Read the model definition and answer for the solid it produces. Units are mm, in the model's axes. Face numbers are marked on the shaded views. Coordinates: 2 decimals unless noted, no trailing zeros. Loops run counter-clockwise (first coordinate to the right, second up) from the corner with the lowest first, then second, coordinate; pieces in that order, holes last.
Q1. Section B-B (x = -25.4) is taken. Give the vertices of the cut face in (y, z).
Q2. Section C-C (y = 4.75) is taken. Give the vertices of the cut face in (x, z) (3 decimals), then the cut area to 3 significant figures.
Q3. Straight lines are drawn through the part: line 1 (Z direction, x = 0, y = 1.25); line 2 (Z direction, x = -25, y = 0); line 3 (X direction, y = -1, z = -16.5). For each, find the intervals that lie inside material, in ascending order.
Q4. The mould has two halves that part along X. Classify the marked faces 1, 2 and 3: pulls with the +X half, pulls with the -X half, needs draft (parallel to the pull), parting line crosses it, or undercut.
Q5. Flat-ended cylindrical pins translate along their axes: P1, Ø7.5, axis at x = -24.892, z = 0, coming from the +Y side; P2, Ø2, axis at y = 2.5, z = -4, coming from the +X side. Find the tip coordinate at first contact, or state that the pin passes through.
Q6. Section A-A (z = 2) is taken. Give the vertices of the cut face in (x, y).
from build123d import *

# Parameters (mm, degrees)
F0_W        = 88.9
F0_H        = 63.5
F0_R        = 3.175
F1_DEPTH    = 6.35
F2_R        = 3.81
F3_DEPTH    = 25.4
F4_T1_DEPTH = 88.9
F4_T3_DEPTH = 114.3


# Not quite as in the source:
# - a fillet or chamfer that OpenCascade refuses, or shapes differently, is made with other operations: its cross-section is extruded or revolved along the edge and cut away or added


with BuildPart() as f1:
    # F0 (on Front) → F1 (new body, symmetric)
    with BuildSketch(Plane.XZ):
        Rectangle(F0_W, F0_H)
        with Locations((0, -24.892)):
            Circle(F0_R, mode=Mode.SUBTRACT)
        with BuildLine():
            ThreePointArc((-21.717, 0), (-24.892, -3.175), (-28.067, 0))
            ThreePointArc((-28.067, 0), (-24.892, 3.175), (-21.717, 0))
        make_face(mode=Mode.SUBTRACT)
        with Locations((24.892, 0)):
            Circle(F0_R, mode=Mode.SUBTRACT)
        with BuildLine():
            ThreePointArc((0, 21.717), (-3.175, 24.892), (0, 28.067))
            ThreePointArc((0, 28.067), (2.2450640303, 27.1370640303), (3.175, 24.892))
            ThreePointArc((3.175, 24.892), (2.2450640303, 22.6469359697), (0, 21.717))
        make_face(mode=Mode.SUBTRACT)
    extrude(amount=F1_DEPTH, both=True)

    # F2 (on face) → F3 (cut)
    with BuildSketch(Plane(origin=(0, 0, -31.75), x_dir=(1, 0, 0), z_dir=(0, 0, -1))):
        with Locations((-25.4, 0)):
            Circle(F2_R)
        with BuildLine():
            ThreePointArc((29.21, 0), (25.4, 3.81), (21.59, 0))
            ThreePointArc((21.59, 0), (25.4, -3.81), (29.21, 0))
        make_face()
    extrude(amount=-F3_DEPTH, mode=Mode.SUBTRACT)

    # F4: fillet of radius 5.08 on 6 edges, made by hand

    # F4_s2 → F4_t1 (cut)
    with BuildSketch(Plane.XY.offset(-44.45)):
        with BuildLine():
            ThreePointArc((-44.45, -1.27), (-42.9621024484, -4.8621024484), (-39.37, -6.35))
            Line((-39.37, -6.35), (-44.45, -6.35))
            Line((-44.45, -6.35), (-44.45, -1.27))
        make_face()
        with BuildLine():
            ThreePointArc((44.45, -1.27), (42.9621024484, -4.8621024484), (39.37, -6.35))
            Line((39.37, -6.35), (44.45, -6.35))
            Line((44.45, -6.35), (44.45, -1.27))
        make_face()
        with BuildLine():
            ThreePointArc((39.37, 6.35), (42.9621024484, 4.8621024484), (44.45, 1.27))
            Line((44.45, 1.27), (44.45, 6.35))
            Line((44.45, 6.35), (39.37, 6.35))
        make_face()
        with BuildLine():
            ThreePointArc((-39.37, 6.35), (-42.9621024484, 4.8621024484), (-44.45, 1.27))
            Line((-44.45, 1.27), (-44.45, 6.35))
            Line((-44.45, 6.35), (-39.37, 6.35))
        make_face()
    extrude(amount=F4_T1_DEPTH, mode=Mode.SUBTRACT)

    # F4_s4 → F4_t3 (cut)
    with BuildSketch(Plane.YZ.offset(-57.15)):
        with BuildLine():
            ThreePointArc((-6.35, 26.67), (-4.8621024484, 30.2621024484), (-1.27, 31.75))
            Line((-1.27, 31.75), (-6.35, 31.75))
            Line((-6.35, 31.75), (-6.35, 26.67))
        make_face()
        with BuildLine():
            ThreePointArc((6.35, 26.67), (4.8621024484, 30.2621024484), (1.27, 31.75))
            Line((1.27, 31.75), (6.35, 31.75))
            Line((6.35, 31.75), (6.35, 26.67))
        make_face()
    extrude(amount=F4_T3_DEPTH, mode=Mode.SUBTRACT)


solid = f1.part
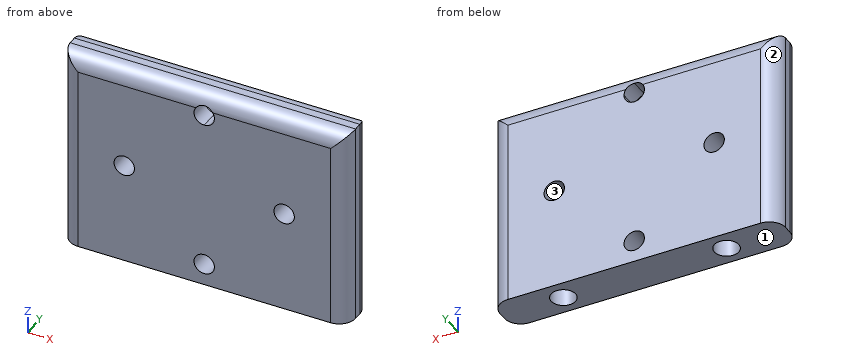
Numbers:
1. outline: (-6.35, -31.75) - (-3.81, -31.75) - (-3.81, -6.35) - (3.81, -6.35) - (3.81, -31.75) - (6.35, -31.75) - (6.35, -3.13) - (-6.35, -3.13) - close; (-6.35, 3.13) - (6.35, 3.13) - (6.35, 26.67) arc R5.08 ccw to (1.27, 31.75) - (-1.27, 31.75) arc R5.08 ccw to (-6.35, 26.67) - close
2. outline: (-43.071, -31.75) - (43.071, -31.75) - (43.071, 30.371) - (-43.071, 30.371) - close; hole circle Ø6.35 at (-24.892, 0); hole circle Ø6.35 at (0, -24.892); hole circle Ø6.35 at (0, 24.892); hole circle Ø6.35 at (24.892, 0)
2. area: 5,220 mm2
3. line 1: z = -31.75 to -28.07, -21.72 to 21.72, 28.07 to 31.75
3. line 2: z = -6.35 to -3.17, 3.17 to 31.75
3. line 3: x = -44.45 to -29.08, -21.72 to 21.72, 29.08 to 44.45
4. face 1: needs draft
4. face 2: pulls with the -X half
4. face 3: undercut
5. P1: stops at y = 6.35
5. P2: stops at x = 44.44
6. outline: (-44.45, -1.27) arc R5.08 ccw to (-39.37, -6.35) - (-27.36, -6.35) - (-27.36, 6.35) - (-39.37, 6.35) arc R5.08 ccw to (-44.45, 1.27) - close; (-22.43, -6.35) - (22.43, -6.35) - (22.43, 6.35) - (-22.43, 6.35) - close; (27.36, -6.35) - (39.37, -6.35) arc R5.08 ccw to (44.45, -1.27) - (44.45, 1.27) arc R5.08 ccw to (39.37, 6.35) - (27.36, 6.35) - close
